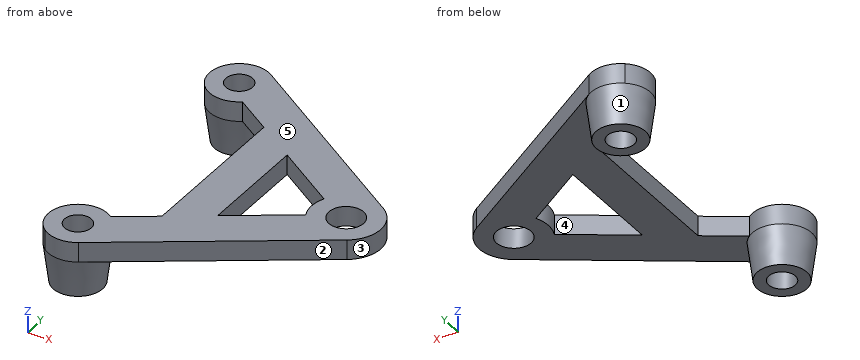
from build123d import *
from build123d.topology import SkipClean

# Parameters (mm, degrees)
SKETCH_1_R          = 2.2
SKETCH_1_R_2        = 2.7
SKETCH_1_R_3        = 3.5
EXTRUDE_1_DEPTH     = 4
SKETCH_5_R          = 2.2
CUT_EXTRUDE_1_DEPTH = 57.443688753


with BuildPart() as part:
    # Sketch 1 → Extrude 1 (new body)
    with BuildSketch(Plane.XY):
        with BuildLine():
            Line((-22.796873936, 30.645831284), (-45, 12.5))
            Line((-45, 12.5), (-45, -12.5))
            Line((-45, -12.5), (-22.796873936, -30.645831284))
            ThreePointArc((-22.796873936, -30.645831284), (-19.320397567, -31.991439343), (-15.720242852, -31.024260448))
            Line((-15.720242852, -31.024260448), (22.82638334, -5.861637189))
            ThreePointArc((22.82638334, -5.861637189), (26, 0), (22.82638334, 5.861637189))
            Line((22.82638334, 5.861637189), (-15.720242852, 31.024260448))
            ThreePointArc((-15.720242852, 31.024260448), (-19.320397567, 31.991439343), (-22.796873936, 30.645831284))
        make_face()
        with Locations((-19, 0)):
            Circle(SKETCH_1_R, mode=Mode.SUBTRACT)
        with Locations((-35, 0)):
            Circle(SKETCH_1_R, mode=Mode.SUBTRACT)
        with Locations((-19, 26)):
            Circle(SKETCH_1_R_2, mode=Mode.SUBTRACT)
        with Locations((-19, -26)):
            Circle(SKETCH_1_R_2, mode=Mode.SUBTRACT)
        with Locations((19, 0)):
            Circle(SKETCH_1_R_3, mode=Mode.SUBTRACT)
    extrude(amount=EXTRUDE_1_DEPTH)

    # Sketch 4 → Revolve 1 (revolve)
    with BuildSketch(Plane(origin=(-25.223829861, 16.46571414, 0), x_dir=(0, 0, -1), z_dir=(0.8373767412950733, -0.5466261914124163, 0)), mode=Mode.PRIVATE) as revolve_1_sk:
        Polygon((7.7, 16.385897637), (0, 17.385897637), (0, 14.085897637), (7.7, 14.085897637), align=None)
    revolve_1 = revolve(revolve_1_sk.sketch.rotate(Axis((-19, 26, 1000.278995542), (0, 0, -1)), 56.864137938), axis=Axis((-19, 26, 1000.278995542), (0, 0, -1)))

    # Mirror 1: Revolve 1 across plane
    add(revolve_1.mirror(Plane.ZX))

    # Sketch 5 → Cut-Extrude 1 (cut, through all)
    # profile 1 of 2: a face of its own
    with SkipClean():  # the faces are left unmerged after this step: merging them gives an invalid solid
        with BuildSketch(Plane.XY.offset(4)):
            with BuildLine():
                Line((-8, 16.430964093), (-15.356334205, 21.233061824))
                ThreePointArc((-15.356334205, 21.233061824), (-23.707008117, 22.279237365), (-22.796873936, 30.645831284))
                Line((-22.796873936, 30.645831284), (-45, 12.5))
                Line((-45, 12.5), (-45, -12.5))
                Line((-45, -12.5), (-22.796873936, -30.645831284))
                ThreePointArc((-22.796873936, -30.645831284), (-23.707008117, -22.279237365), (-15.356334205, -21.233061824))
                Line((-15.356334205, -21.233061824), (-8, -16.430964093))
                Line((-8, -16.430964093), (-8, 16.430964093))
            make_face()
            with Locations((-35, 0)):
                Circle(SKETCH_5_R, mode=Mode.SUBTRACT)
            with Locations((-19, 0)):
                Circle(SKETCH_5_R, mode=Mode.SUBTRACT)
        # profile 2 of 2: a face of its own
        with BuildSketch(Plane.XY.offset(4)):
            with BuildLine():
                Line((12.651857565, 2.949760604), (0, 11.208691589))
                Line((0, 11.208691589), (0, -11.208691589))
                Line((0, -11.208691589), (12.651857565, -2.949760604))
                ThreePointArc((12.651857565, -2.949760604), (12, 0), (12.651857565, 2.949760604))
            make_face()
        extrude(amount=-CUT_EXTRUDE_1_DEPTH, mode=Mode.SUBTRACT)


solid = part.part
The listing builds one solid part. Answer for the finished solid, in the listing's coordinates (mm). Face numbers are marked on the shaded views. A direction names the side the tool comes from. Round coordinates to 2 decimals unless told otherwise and drop trailing zeros. Write each loop counter-clockwise with the first axis right and the second up, starting at its lowest first coordinate (ties: lowest second). Pieces come first, ordered by that corner, then holes. Notation, with made-up numbers: M -35.5,14.5 L 20.5,14.5 A17 cw 20.5,42.5 Z; hole C -39,9 d2. An arc over 180 degrees is marked long. Write each question's results on one line, items separated by ' | '. Start each with the question number.
Item 1: Which of the six approach directions +Z, -Z, +X, -X, +Y, -Y give full straight-line access (tool end or side, diameter ignored) to the marked faces 4 and 5?
Item 2: Given pin 1 Ø5 at (x, y) = (-19, -26) entering from -Z; pin 2 Ø3 at (x, y) = (2, 15.5) entering from -Z; pin 3 Ø5 at (x, z) = (4, -1) entering from +Y; pin 4 Ø1.5 at (x, z) = (-16, 1) entering from -Y, each flat-ended and moving along its own axis, determine where each tip first touches the part or whether it passes through.
Item 3: Straight lines are drawn through the part: probe 1 along Y at (x, z) = (-19, 1); probe 2 along Y at (x, z) = (-19, -2); probe 3 along Z at (x, y) = (13.5, -2). For each, find the intervals that lie inside material, in ascending order.
Item 4: Find section C-C on z = 3. Write down the section's boundary in (x, y).
Item 5: The mould has two halves that part along Y. Classify the marked faces 1, 2 and 3: +Y half, -Y half, draft (parallel to the pull), parting line (faces both ways), or undercut.
Item 6: Find section A-A on x = -19. Write down the section's boundary in (y, z), and give its area (3 significant figures).
Item 7: Find section D-D on x = 10.5. Write down the section's boundary in (y, z).
Item 8: Find section B-B on y = 26. Write down the section's boundary in (x, z).
Answer block:
1) face 4: +Z, -Z | face 5: +Z, +X, -X, +Y, -Y
2) pin 1: passes through | pin 2: stops at z = 0 | pin 3: stops at y = 19.65 | pin 4: stops at y = -31.56
3) probe 1: y = -32 to -28.7, -23.3 to -20, 20 to 23.3, 28.7 to 32 | probe 2: y = -31.74 to -28.7, -23.3 to -20.26, 20.26 to 23.3, 28.7 to 31.74 | probe 3: z = 0 to 4
4) outline: M -15.72,-31.02 L 22.83,-5.86 A7 ccw 22.83,5.86 L -15.72,31.02 A6 ccw long -15.36,21.23 L -8,16.43 L -8,-16.43 L -15.36,-21.23 A6 ccw long Z; hole C -19,-26 d5.4; hole C -19,26 d5.4; hole M 0,-11.21 L 12.65,-2.95 A7 cw 12.65,2.95 L 0,11.21 Z; hole C 19,0 d7
5) face 1: undercut | face 2: -Y half | face 3: parting line
6) outline: M -32,0 L -31,-7.7 L -28.7,-7.7 L -28.7,4 L -32,4 Z; M -23.3,-7.7 L -21,-7.7 L -20,0 L -20,4 L -23.3,4 Z; M 20,0 L 21,-7.7 L 23.3,-7.7 L 23.3,4 L 20,4 Z; M 28.7,-7.7 L 31,-7.7 L 32,0 L 32,4 L 28.7,4 Z | area: 139 mm²
7) outline: M -13.91,0 L -4.35,0 L -4.35,4 L -13.91,4 Z; M 4.35,0 L 13.91,0 L 13.91,4 L 4.35,4 Z
8) outline: M -25,0 L -24,-7.7 L -21.7,-7.7 L -21.7,4 L -25,4 Z; M -16.3,-7.7 L -14,-7.7 L -13,0 L -8.02,0 L -8.02,4 L -16.3,4 Z
